Autodesk Inventor part; units mm, degrees
ref_plane "YZ Plane" through (0, 0, 0) normal (1, 0, 0) x (0, 1, 0)
ref_plane "XZ Plane" through (0, 0, 0) normal (0, 1, 0) x (-1, 0, 0)
ref_plane "XY Plane" through (0, 0, 0) normal (0, 0, 1) x (1, 0, 0)
sketch "Skizze1" plane through (0, 0, 0) normal (0, 1, 0) x (-1, 0, 0)
  line L0 (0, 0) -> (-45.5, 0) construction
  line L1 (-45.5, 0) -> (-45.5, -48) construction
  line L2 (-45.5, -48) -> (0, -48) construction
  line L3 (0, -48) -> (0, 0) construction
  circle A0 centre (-4, -36.5) radius 1.75
  circle A1 centre (-42.5, -36.5) radius 1.75
  circle A2 centre (-27.95, -4) radius 1.75
  line L4 (5, -53) -> (-50.5, -53)
  line L5 (-50.5, -53) -> (-50.5, 5)
  line L6 (-50.5, 5) -> (5, 5)
  line L7 (5, 5) -> (5, -53)
  dimension "d0" = 45.5
  dimension "d1" = 48
  dimension "d2" = 11.5
  dimension "d3" = 11.5
  dimension "d4" = 3
  dimension "d5" = 4
  dimension "d6" = 17.55
  dimension "d7" = 4
  dimension "d8" = 3.5
  dimension "d9" = 5
  dimension "d10" = 5
  dimension "d11" = 5
  dimension "d12" = 5
extrude "Extrusion1" add sketch "Skizze1" along normal blind 3
properties part number "Sensor_Schutzplatte"
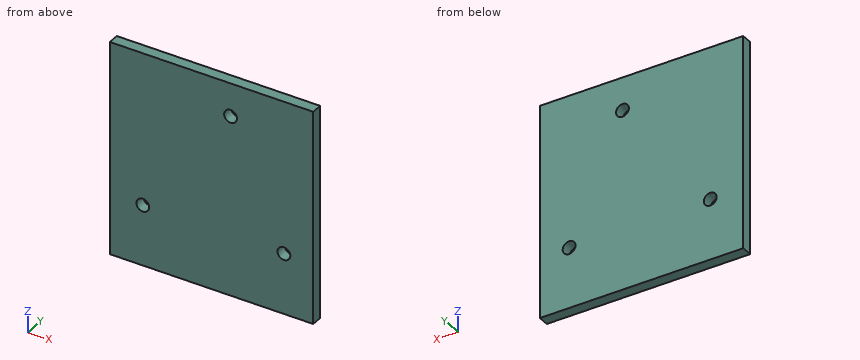
The model under review builds one solid part; all positions refer to its coordinate system, in mm. Give positions to 0.01 mm unless a question says otherwise; leave off trailing zeros. Write each loop counter-clockwise with the first axis right and the second up, starting at its lowest first coordinate (ties: lowest second). Pieces come first, ordered by that corner, then holes.
(1) To check wall thickness, follow L1, parallel to X at y = 1.1, z = -36; L2, parallel to Z at x = 4, y = 0.65; L3, parallel to Z at x = 27.95, y = 1.9. State the ranges of each line that lie inside material, in increasing order.
(2) For P1, Ø3, axis at x = 27.95, z = -4, coming from the +Y side, flat-tipped, find the tip position at first contact; note if it passes through.
(3) Consider section A-A, the plane x = 27.95. Give the boundary of the cut face in (y, z).
(4) Consider section B-B, the plane z = -4. Give the boundary of the cut face in (x, y).
Returned:
1. L1: x = -5 to 2.32, 5.68 to 40.82, 44.18 to 50.5
1. L2: z = -53 to -38.25, -34.75 to 5
1. L3: z = -53 to -5.75, -2.25 to 5
2. P1: passes through
3. outline: (0, -53) - (3, -53) - (3, -5.75) - (0, -5.75) - close; (0, -2.25) - (3, -2.25) - (3, 5) - (0, 5) - close
4. outline: (-5, 0) - (26.2, 0) - (26.2, 3) - (-5, 3) - close; (29.7, 0) - (50.5, 0) - (50.5, 3) - (29.7, 3) - close
